```python
from build123d import *

# Parameters (mm, degrees)
SKETCH_R     = 0.95
SKETCH_R_2   = 0.55
PAD_DEPTH    = 1
SKETCH001_W  = 10
SKETCH001_H  = 10
PAD001_DEPTH = 4
SKETCH002_W  = 2
SKETCH002_H  = 1
PAD002_DEPTH = 0.5
SKETCH006_W  = 9.5
SKETCH006_H  = 8
PAD006_DEPTH = 3


with BuildPart() as part:
    # Sketch → Pad (new body)
    with BuildSketch(Plane.XY):
        Polygon((-36, -13.5), (36, -13.5), (36, 13.5), (-34.090812, 13.5), (-36, 11.590812), align=None)
        with Locations((-34.25, 10.65)):
            Circle(SKETCH_R, mode=Mode.SUBTRACT)
        with Locations((33.85, -7.55)):
            Circle(SKETCH_R, mode=Mode.SUBTRACT)
        with Locations((33.85, -10.75)):
            Circle(SKETCH_R, mode=Mode.SUBTRACT)
        with Locations((-2.45, 11.45)):
            Circle(SKETCH_R, mode=Mode.SUBTRACT)
        with Locations((-29.45, -11.25)):
            Circle(SKETCH_R_2, mode=Mode.SUBTRACT)
        with Locations((17.95, -11.25)):
            Circle(SKETCH_R_2, mode=Mode.SUBTRACT)
    extrude(amount=-PAD_DEPTH)

    # Sketch001 (on Face12 of Pad) → Pad001 (join)
    with BuildSketch(Plane.XY):
        with Locations((-19.4, -7)):
            Rectangle(SKETCH001_W, SKETCH001_H)
    extrude(amount=PAD001_DEPTH)

    # Sketch002 (on Face5 of Pad001) → Pad002 (join)
    with BuildSketch(Plane(origin=(0, 0, -1), x_dir=(1, 0, 0), z_dir=(0, 0, -1))):
        with Locations((-27, 7.5)):
            Rectangle(SKETCH002_W, SKETCH002_H)
        with Locations((-27, 4.3)):
            Rectangle(SKETCH002_W, SKETCH002_H)
        with Locations((-27, 1.4)):
            Rectangle(SKETCH002_W, SKETCH002_H)
        with Locations((-27, -1.5)):
            Rectangle(SKETCH002_W, SKETCH002_H)
        with Locations((-27, -4)):
            Rectangle(SKETCH002_W, SKETCH002_H)
    extrude(amount=PAD002_DEPTH)

    # Sketch006 (on Face4 of Pad002) → Pad006 (join)
    with BuildSketch(Plane.XY):
        with Locations((-26.25, 11.5)):
            Rectangle(SKETCH006_W, SKETCH006_H)
    extrude(amount=PAD006_DEPTH)


solid = part.part
```
Check sheet for the modelled part. Datum: model origin and axes. Units: mm. A direction names the side the tool comes from. Round coordinates to 2 decimals unless told otherwise and drop trailing zeros. Order: outer loops, then holes, each group sorted by start corner. A loop starts at its lowest first (then second) coordinate and runs counter-clockwise, first axis right, second up.
1) Scan lines: line 1 (Y direction, x = 33.85, z = -0.3); line 2 (Y direction, x = 17.95, z = -0.25); line 3 (Z direction, x = -6, y = -10.25). Record each from-to range of solid material in increasing order.
2) Section check A-A (x = -2.45). Record the boundary of the cut face in (y, z).
3) Section check C-C (x = 33.85). Record the boundary of the cut face in (y, z).
4) Go/stop test with flat-tipped pins: pin 1 Ø0.6 at (x, z) = (-26.5, -1.5) entering from -Y; pin 2 Ø12 at (x, y) = (1, 12.5) entering from -Z; pin 3 Ø8 at (x, y) = (-9.5, 6.5) entering from +Z; pin 4 Ø1.7 at (x, y) = (33.85, -10.75) entering from -Z. Record where each tip stops, or that it passes through.
5) Tool access check on faces 1 (the flat face through (-14.4, -7, 2)), 2 (the flat face through (-26, 7.5, 1)), 3 (the flat face through (-31, 11, 1)), 4 (the flat face through (-26, 12, 3)), 5 (the flat face through (-24.4, -7, 2)). Record the directions out of +Z, -Z, +X, -X, +Y, -Y that give a thin tool (end or side, any length) a straight path to the whole face; none if there is none.
6) Section check B-B (z = 1.05). Record the boundary of the cut face in (x, y).
7) Section check D-D (y = -3). Record the boundary of the cut face in (x, z).
8) Mould release check, pull along X, two halves, no side actions. Record for faces 6 (the flat face through (-21.5, 11, 1)), 7 (the cylindrical face through (33.726, -9.808, -0.493)), 8 (the flat face through (-19, -2, 2)): +X half, -X half, draft (parallel to the pull), parting line (faces both ways), or undercut.
Result:
1. line 1: y = -13.5 to -11.7, -9.8 to -8.5, -6.6 to 13.5
1. line 2: y = -13.5 to -11.8, -10.7 to 13.5
1. line 3: z = -1 to 0
2. outline: (-13.5, -1) - (10.5, -1) - (10.5, 0) - (-13.5, 0) - close; (12.4, -1) - (13.5, -1) - (13.5, 0) - (12.4, 0) - close
3. outline: (-13.5, -1) - (-11.7, -1) - (-11.7, 0) - (-13.5, 0) - close; (-9.8, -1) - (-8.5, -1) - (-8.5, 0) - (-9.8, 0) - close; (-6.6, -1) - (13.5, -1) - (13.5, 0) - (-6.6, 0) - close
4. pin 1: stops at y = -8
4. pin 2: stops at z = -1
4. pin 3: stops at z = 0
4. pin 4: passes through
5. face 1: +Z, +X, +Y, -Y
5. face 2: +Z, +X, -X
5. face 3: +Z, -X, +Y, -Y
5. face 4: +Z, +X, -X, +Y
5. face 5: +Z, -X, -Y
6. outline: (-31, 7.5) - (-21.5, 7.5) - (-21.5, 15.5) - (-31, 15.5) - close; (-24.4, -12) - (-14.4, -12) - (-14.4, -2) - (-24.4, -2) - close
7. outline: (-36, -1) - (36, -1) - (36, 0) - (-14.4, 0) - (-14.4, 4) - (-24.4, 4) - (-24.4, 0) - (-36, 0) - close
8. face 6: +X half
8. face 7: undercut
8. face 8: draft
